Source: CAD feature listing. Evaluate the final solid. Frame: model axes, mm. Give positions to 0.01 mm unless a question says otherwise; leave off trailing zeros. Order: outer loops, then holes, each group sorted by start corner. A loop starts at its lowest first (then second) coordinate and runs counter-clockwise, first axis right, second up. Notation, with made-up numbers: M -37,-23.5 L -25,-23.5 A36 ccw -25,11.5 Z; hole C 83,-26 d2. An arc over 180 degrees is marked long. Use CSV: the item, a comma, the result in double quotes. Start each with the question number.
1. Section query A-A, the plane x = 1.4. Return the cut outline in (y, z), plus the area to 3 significant figures.
2. Pin query (flat end, axial travel): P1, Ø1.6, axis at y = 0, z = -7.24, coming from the +X side; P2, Ø0.9, axis at x = 1, y = 3.5, coming from the +Z side; P3, Ø1.5, axis at x = 0.5, y = -11.5, coming from the -Z side; P4, Ø1, axis at x = 2, y = -3, coming from the -Z side. Return the tip coordinate at first contact, or that it passes through.
3. Line query: line 1 along Y through (x, z) = (1.2, 0); line 2 along Y through (x, z) = (0.6, 7.24); line 3 along Z through (x, y) = (0.45, -12). Output: solid intervals per line, ascending. Write a range as [from, to].
4. Section query C-C, the plane z = -7.24. Return the cut outline in (x, y).
5. Section query D-D, the plane z = 2. Return the cut outline in (x, y).
6. Section query B-B, the plane y = 0. Return the cut outline in (x, z).
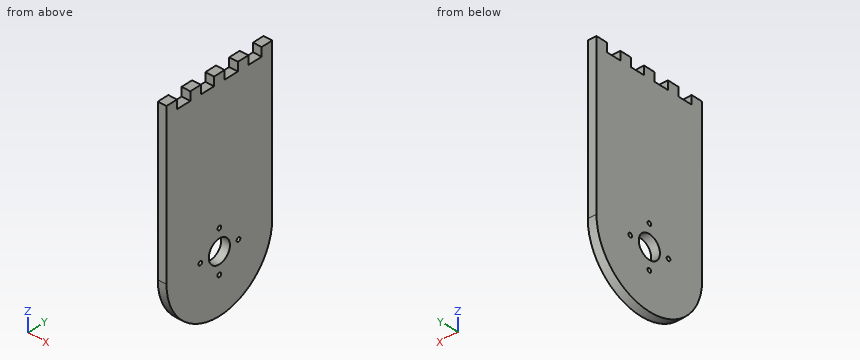
from build123d import *

# Parameters (mm, degrees)
SKETCH1_R           = 4
SKETCH1_R_2         = 0.7
BOSS_EXTRUDE1_DEPTH = 3


with BuildPart() as part:
    # Sketch1 → Boss-Extrude1 (new body)
    with BuildSketch(Plane(origin=(0, 0, 0), x_dir=(0, 0, -1), z_dir=(1, 0, 0))):
        with BuildLine():
            Line((0, 20), (-55, 20))
            Line((-55, 20), (-55, 16))
            Line((-55, 16), (-52, 16))
            Line((-52, 16), (-52, 11))
            Line((-52, 11), (-55, 11))
            Line((-55, 11), (-55, 7))
            Line((-55, 7), (-52, 7))
            Line((-52, 7), (-52, 2))
            Line((-52, 2), (-55, 2))
            Line((-55, 2), (-55, -2))
            Line((-55, -2), (-52, -2))
            Line((-52, -2), (-52, -7))
            Line((-52, -7), (-55, -7))
            Line((-55, -7), (-55, -11))
            Line((-55, -11), (-52, -11))
            Line((-52, -11), (-52, -16))
            Line((-52, -16), (-55, -16))
            Line((-55, -16), (-55, -20))
            Line((-55, -20), (0, -20))
            ThreePointArc((0, -20), (20, 0), (0, 20))
        make_face()
        Circle(SKETCH1_R, mode=Mode.SUBTRACT)
        with Locations((-7.24, 0)):
            Circle(SKETCH1_R_2, mode=Mode.SUBTRACT)
        with Locations((0, 7.24)):
            Circle(SKETCH1_R_2, mode=Mode.SUBTRACT)
        with Locations((7.24, 0)):
            Circle(SKETCH1_R_2, mode=Mode.SUBTRACT)
        with Locations((0, -7.24)):
            Circle(SKETCH1_R_2, mode=Mode.SUBTRACT)
    extrude(amount=BOSS_EXTRUDE1_DEPTH)


solid = part.part
Result set:
1,outline,"M -20,0 A20 ccw 20,0 L 20,55 L 16,55 L 16,52 L 11,52 L 11,55 L 7,55 L 7,52 L 2,52 L 2,55 L -2,55 L -2,52 L -7,52 L -7,55 L -11,55 L -11,52 L -16,52 L -16,55 L -20,55 Z; hole C -7.24,0 d1.4; hole C 0,0 d8; hole C 0,-7.24 d1.4; hole C 0,7.24 d1.4; hole C 7.24,0 d1.4"
1,area,"2,710 mm2"
2,P1,"x = 3"
2,P2,"z = 52"
2,P3,"z = -16.87"
2,P4,"z = -19.84"
3,line 1,"[-20, -7.94], [-6.54, -4], [4, 6.54], [7.94, 20]"
3,line 2,"[-20, -0.7], [0.7, 20]"
3,line 3,"[-16, 52]"
4,outline,"M 0,-18.64 L 3,-18.64 L 3,-0.7 L 0,-0.7 Z; M 0,0.7 L 3,0.7 L 3,18.64 L 0,18.64 Z"
5,outline,"M 0,-20 L 3,-20 L 3,-3.46 L 0,-3.46 Z; M 0,3.46 L 3,3.46 L 3,20 L 0,20 Z"
6,outline,"M 0,-20 L 3,-20 L 3,-7.94 L 0,-7.94 Z; M 0,-6.54 L 3,-6.54 L 3,-4 L 0,-4 Z; M 0,4 L 3,4 L 3,6.54 L 0,6.54 Z; M 0,7.94 L 3,7.94 L 3,55 L 0,55 Z"
